```python
from build123d import *

# Parameters (mm, degrees)
SKETCH3_R           = 2
BOSS_EXTRUDE1_DEPTH = 5.2
SKETCH4_R           = 2
BOSS_EXTRUDE2_DEPTH = 8.6
SKETCH5_R           = 2
BOSS_EXTRUDE3_DEPTH = 15
SKETCH7_R           = 2
BOSS_EXTRUDE4_DEPTH = 6
SKETCH8_R           = 10
BOSS_EXTRUDE5_DEPTH = 2.5
CUT_EXTRUDE1_DEPTH  = 12


with BuildPart() as part:
    # Sketch3 → Boss-Extrude1 (new body)
    with BuildSketch(Plane.XY):
        Circle(SKETCH3_R)
    extrude(amount=BOSS_EXTRUDE1_DEPTH)

    # Sketch4 → Boss-Extrude2 (add)
    with BuildSketch(Plane.XY.offset(5.2)):
        with Locations(Location((0, 0, 0), (0, 0, 119))):
            Circle(SKETCH4_R)
        with BuildLine():
            Line((0, 0), (1.139302608, 2.055356312))
            ThreePointArc((1.139302608, 2.055356312), (0, 2.35), (-1.139302608, 2.055356312))
            Line((-1.139302608, 2.055356312), (0, 0))
        make_face()
        with BuildLine():
            Line((0.96961924, 1.749239414), (0, 0))
            Line((0, 0), (-0.96961924, 1.749239414))
            ThreePointArc((-0.96961924, 1.749239414), (-1.015076726, -1.723258321), (2, 0))
            ThreePointArc((2, 0), (1.723258321, 1.015076726), (0.96961924, 1.749239414))
        make_face()
    extrude(amount=BOSS_EXTRUDE2_DEPTH)

    # Sketch5 → Boss-Extrude3 (add)
    with BuildSketch(Plane.XY.offset(13.8)):
        Circle(SKETCH5_R)
    extrude(amount=BOSS_EXTRUDE3_DEPTH)

    # Sketch7 → Boss-Extrude4 (add)
    with BuildSketch(Plane.XY.offset(28.8)):
        Circle(SKETCH7_R)
    extrude(amount=BOSS_EXTRUDE4_DEPTH)

    # Sketch8 → Boss-Extrude5 (add)
    with BuildSketch(Plane.XY.offset(34.8)):
        Circle(SKETCH8_R)
    extrude(amount=BOSS_EXTRUDE5_DEPTH)

    # Sketch9 → Cut-Extrude1 (cut)
    with BuildSketch(Plane.XY.offset(37.3)):
        with BuildLine():
            Line((7.509902395, -2.992467491), (3.464101615, -2))
            Line((3.464101615, -2), (6.346504065, -5.007532509))
            ThreePointArc((6.346504065, -5.007532509), (7.935735739, -4.581699165), (7.509902395, -2.992467491))
        make_face()
        with BuildLine():
            Line((-6.346504065, 5.007532509), (-3.464101615, 2))
            Line((-3.464101615, 2), (-7.509902395, 2.992467491))
            ThreePointArc((-7.509902395, 2.992467491), (-7.935735739, 4.581699165), (-6.346504065, 5.007532509))
        make_face()
        with BuildLine():
            Line((-7.509902395, -2.992467491), (-3.464101615, -2))
            Line((-3.464101615, -2), (-6.346504065, -5.007532509))
            ThreePointArc((-6.346504065, -5.007532509), (-7.935735739, -4.581699165), (-7.509902395, -2.992467491))
        make_face()
        with BuildLine():
            Line((6.346504065, 5.007532509), (3.464101615, 2))
            Line((3.464101615, 2), (7.509902395, 2.992467491))
            ThreePointArc((7.509902395, 2.992467491), (7.935735739, 4.581699165), (6.346504065, 5.007532509))
        make_face()
        with BuildLine():
            Line((-1.16339833, -8), (0, -4))
            Line((0, -4), (1.16339833, -8))
            ThreePointArc((1.16339833, -8), (0, -9.16339833), (-1.16339833, -8))
        make_face()
        with BuildLine():
            Line((1.16339833, 8), (0, 4))
            Line((0, 4), (-1.16339833, 8))
            ThreePointArc((-1.16339833, 8), (0, 9.16339833), (1.16339833, 8))
        make_face()
        with BuildLine():
            Line((-8, 1.16339833), (-4, 0))
            Line((-4, 0), (-8, -1.16339833))
            ThreePointArc((-8, -1.16339833), (-9.16339833, 0), (-8, 1.16339833))
        make_face()
        with BuildLine():
            Line((8, -1.16339833), (4, 0))
            Line((4, 0), (8, 1.16339833))
            ThreePointArc((8, 1.16339833), (9.16339833, 0), (8, -1.16339833))
        make_face()
        with BuildLine():
            Line((-2.992467491, 7.509902395), (-2, 3.464101615))
            Line((-2, 3.464101615), (-5.007532509, 6.346504065))
            ThreePointArc((-5.007532509, 6.346504065), (-4.581699165, 7.935735739), (-2.992467491, 7.509902395))
        make_face()
        with BuildLine():
            Line((5.007532509, -6.346504065), (2, -3.464101615))
            Line((2, -3.464101615), (2.992467491, -7.509902395))
            ThreePointArc((2.992467491, -7.509902395), (4.581699165, -7.935735739), (5.007532509, -6.346504065))
        make_face()
        with BuildLine():
            Line((2.992467491, 7.509902395), (2, 3.464101615))
            Line((2, 3.464101615), (5.007532509, 6.346504065))
            ThreePointArc((5.007532509, 6.346504065), (4.581699165, 7.935735739), (2.992467491, 7.509902395))
        make_face()
        with BuildLine():
            Line((-5.007532509, -6.346504065), (-2, -3.464101615))
            Line((-2, -3.464101615), (-2.992467491, -7.509902395))
            ThreePointArc((-2.992467491, -7.509902395), (-4.581699165, -7.935735739), (-5.007532509, -6.346504065))
        make_face()
    extrude(amount=-CUT_EXTRUDE1_DEPTH, mode=Mode.SUBTRACT)


solid = part.part
```
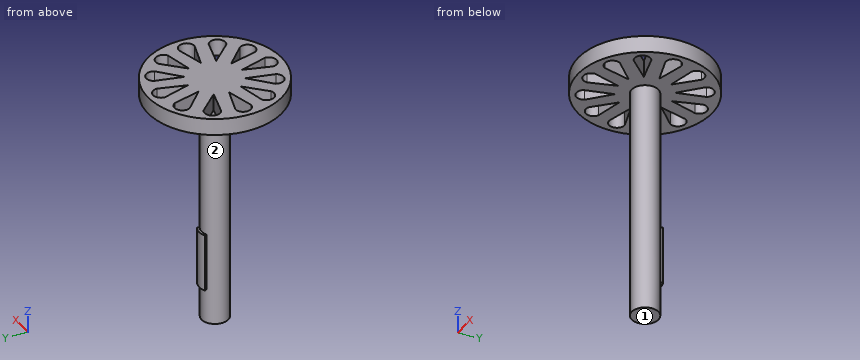
Could you check a few things on this model? Use its own coordinates, in mm. Face numbers are marked on the shaded views. A direction names the side the tool comes from. Round coordinates to 2 decimals unless told otherwise and drop trailing zeros. Loops run counter-clockwise (first coordinate to the right, second up) from the corner with the lowest first, then second, coordinate; pieces in that order, holes last.
Q1. For P1, Ø6, axis at y = -3.5, z = 13, coming from the -X side; P2, Ø4, axis at x = 0.5, z = 11.5, coming from the -Y side; P3, Ø8, axis at y = 3, z = 19, coming from the +X side, each with a flat end and sliding along its axis, tell me the tip position at first contact or that it passes through.
Q2. Please list where these lines run through material, in increasing order: L1, parallel to Z at x = -2, y = 6.5; L2, parallel to X at y = 1.75, z = 32; L3, parallel to Y at x = 1.5, z = 29.
Q3. I want a section at A-A (x = 8.5). Write out the boundary of the cut face in (y, z), and give its area (3 significant figures).
Q4. On a 3-axis mill with a long thin cutter (end or side, diameter ignored), from which of +Z, -Z, +X, -X, +Y, -Y can I reach the whole of each face in a straight line? I mean the marked faces 1 and 2. Say none if no direction works.
Q5. I want a section at B-B (z = 10). Write out the boundary of the cut face in (x, y).
Q6. I want a section at C-C (z = 32). Write out the boundary of the cut face in (x, y), and give its area (3 significant figures).
Answer below:
1. P1: stops at x = -1.94
1. P2: stops at y = -2
1. P3: stops at x = 2
2. L1: z = 34.8 to 37.3
2. L2: x = -0.97 to 0.97
2. L3: y = -1.32 to 1.32
3. outline: (-5.27, 34.8) - (-1.05, 34.8) - (-1.05, 37.3) - (-5.27, 37.3) - close; (1.05, 34.8) - (5.27, 34.8) - (5.27, 37.3) - (1.05, 37.3) - close
3. area: 21.1 mm2
4. face 1: -Z, +X, -X, +Y, -Y
4. face 2: none
5. outline: (-1.14, 2.06) - (-0.97, 1.75) arc R2 ccw (long way) to (0.97, 1.75) - (1.14, 2.06) arc R2.35 ccw to start
6. outline: circle Ø4 at (0, 0)
6. area: 12.6 mm2
